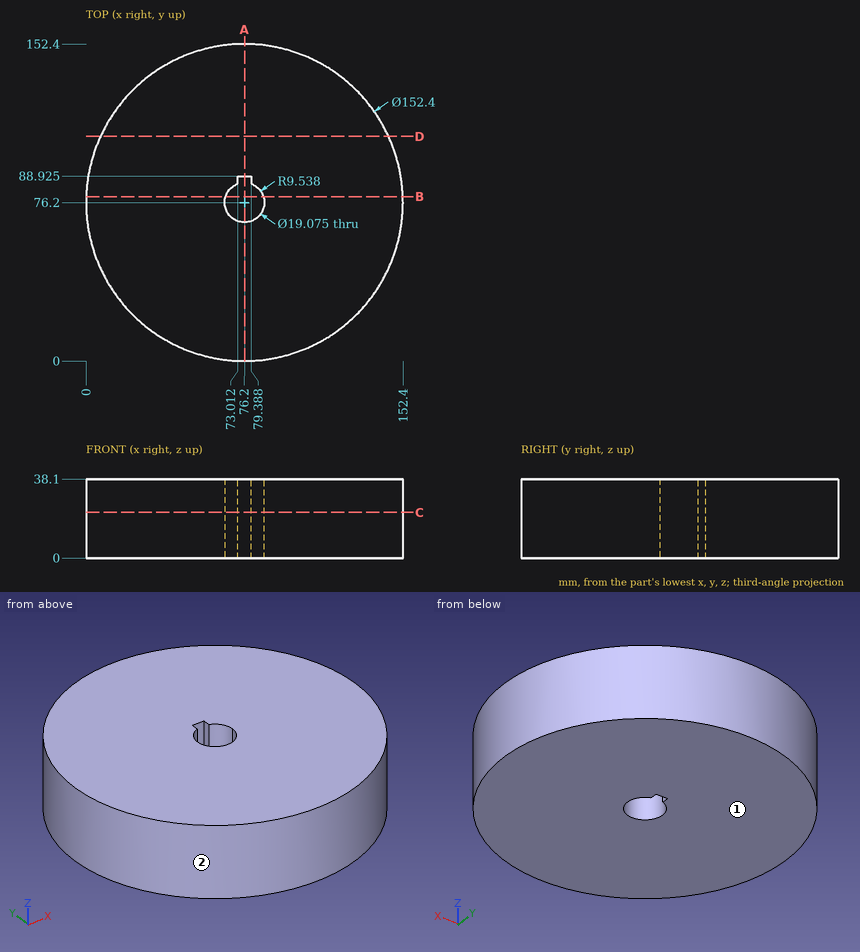
Design review of the part shown in the three views and the two pictorial views. Dimensions are in mm from the part's minimum x, y and z. Round coordinates to 2 decimals unless told otherwise and drop trailing zeros. Write each loop counter-clockwise with the first axis right and the second up, starting at its lowest first coordinate (ties: lowest second). Pieces come first, ordered by that corner, then holes.
Item 1: Draft analysis for pull direction Y (two halves, no side actions). For the marked faces 1 and 2, state which applies: released by +Y, released by -Y, zero draft, split by the parting line, or undercut.
Item 2: Consider section C-C on z = 22. Give the boundary of the cut face in (x, y) (1 decimal), and give its area (3 significant figures).
Item 3: Wall thickness on L1, parallel to Y at x = 76, z = 14 (1 decimal); L2, parallel to X at y = 76.5, z = 29; L3, parallel to Y at x = 68.5, z = 11: over which ranges is each line inside the solid? List them lowest first.
Item 4: For pin 1 Ø2 at (y, z) = (95, 28) entering from +X; pin 2 Ø15.5 at (x, y) = (76.2, 76.2) entering from -Z; pin 3 Ø1.1 at (y, z) = (86.5, 22.5) entering from -X; pin 4 Ø1.5 at (x, y) = (95.5, 74) entering from -Z, all flat-tipped, find the tip position at first contact; note any pin that passes through.
Item 5: Consider section D-D on y = 108. Give the boundary of the cut face in (x, z), and give its area (3 significant figures).
Item 6: Consider section B-B on y = 79. Give the boundary of the cut face in (x, z).
Item 7: Consider section A-A on x = 76.2. Give the boundary of the cut face in (y, z) (1 decimal).
Check values:
1. face 1: zero draft
1. face 2: split by the parting line
2. outline: circle Ø152.4 at (76.2, 76.2); hole (73, 85.2) arc R9.5 ccw (long way) to (79.4, 85.2) - (79.4, 88.9) - (73, 88.9) - close
2. area: 17,900 mm2
3. L1: y = 0 to 66.7, 88.9 to 152.4
3. L2: x = 0 to 66.67, 85.73 to 152.4
3. L3: y = 0.39 to 70.57, 81.83 to 152.01
4. pin 1: stops at x = 150.29
4. pin 2: passes through
4. pin 3: stops at x = 0.63
4. pin 4: stops at z = 0
5. outline: (6.95, 0) - (145.45, 0) - (145.45, 38.1) - (6.95, 38.1) - close
5. area: 5,280 mm2
6. outline: (0.05, 0) - (67.08, 0) - (67.08, 38.1) - (0.05, 38.1) - close; (85.32, 0) - (152.35, 0) - (152.35, 38.1) - (85.32, 38.1) - close
7. outline: (0, 0) - (66.7, 0) - (66.7, 38.1) - (0, 38.1) - close; (88.9, 0) - (152.4, 0) - (152.4, 38.1) - (88.9, 38.1) - close
